Here's how the part is built. I have some questions about the finished solid (model axes, mm). A direction names the side the tool comes from. Round coordinates to 2 decimals unless told otherwise and drop trailing zeros. Write each loop counter-clockwise with the first axis right and the second up, starting at its lowest first coordinate (ties: lowest second). Pieces come first, ordered by that corner, then holes. Notation, with made-up numbers: (36.25, 22.5) -> (41.25, 22.5) arc R22 cw to (41.25, 45.5) -> close; hole circle Ø9 at (61.5, 7.25). An arc over 180 degrees is marked (long way). Put each result on its own line as item: value. Start each with the question number.
1) We'd pull the mould along X, two halves only. Please class faces 1 (the flat face through (27.254, -17, -25)), 2 (the flat face through (11.252, -17, -30)), 3 (the flat face through (31.254, -17, -25)): released by +X, released by -X, zero draft, split by the parting line, or undercut.
2) Which directions (+Z, -Z, +X, -X, +Y, -Y) give clear straight access to the entire face, cutting with the end or side of a thin tool? Please do faces 4 (the flat face through (3.308, -18, -25)), 5 (the flat face through (25.5, -15.6, -28.5)), 6 (the flat face through (7.3, -15.6, -28.5)), 7 (the flat face through (22.36, -17, -25)), 8 (the flat face through (16.678, -17.513, -30.305)).
3) I want a section at A-A, the plane x = 7.5. List the corners of the cut face in (y, z) for me, then the cut area to 3 significant figures.
4) If I drill on line 1 along X through (y, z) = (-17.5, -25.75); line 2 along Y through (x, z) = (23.5, -26.5); line 3 along X through (y, z) = (-18, -25.75), over which ranges is the centre line in solid material (lowest first)? Write a range as [from, to].
5) I want a section at D-D, the plane z = -23. List the corners of the cut face in (x, y) for me.
6) I want a section at C-C, the plane z = -30.25. List the corners of the cut face in (x, y) for me, then the cut area to 3 significant figures.
7) I want a section at B-B, the plane y = -20. List the corners of the cut face in (x, z) for me, then the cut area to 3 significant figures.
8) Will these pins go through, and if not, where does the flat tip stop? P1, Ø1.5, axis at y = -16, z = -30, coming from the -X side; P2, Ø2.5, axis at x = 8.5, y = -16.5, coming from the -Z side; P3, Ø2, axis at x = 16.058, z = -28.5, coming from the -Y side; P4, Ø2.5, axis at y = -16, z = -30.5, coming from the +X side.
Solid Edge part; units mm, degrees
sketch "Sketch1" plane through (0, 0, -22.5) normal (0, 0, 1) x (1, 0, 0)
  line L0 (22.3605, -19.157) -> (22.3605, -15.757)
  line L1 (22.3605, -15.757) -> (27.2537, -15.757)
  line L2 (27.2537, -15.757) -> (27.2537, -19.157)
  line L3 (27.2537, -19.157) -> (22.3605, -19.157)
  line L4 (3.308, -13.457) -> (31.2537, -13.457)
  line L5 (31.2537, -13.457) -> (31.2537, -21.457)
  line L6 (31.2537, -21.457) -> (3.308, -21.457)
  line L7 (3.308, -21.457) -> (3.308, -13.457)
  circle A0 centre (7.308, -17.457) radius 1.7
extrude "ExtrudedProtrusion_1" add sketch "Sketch1" against normal blind 9
sketch "Sketch2" plane through (17.2808, -21.457, -27.5) normal (0, -1, 0) x (0, 0, -1)
  line L0 (2.1809, 0) -> (3.4472, -1.2228)
  line L1 (3.4472, -1.2228) -> (2.1809, -2.4457)
  arc A0 (2.1809, -2.4457) -> (2.1809, 0) centre (1, -1.2228) cw
  dimension "D1" = 1
extrude "Cutout1" cut sketch "Sketch2" against normal up to next
sketch "Sketch3" plane through (17.2808, -17.457, -31.5) normal (0, 0, -1) x (0, 1, 0)
  line L0 (-9.6759, 16.4709) -> (6.2372, 16.4709)
  line L1 (6.2372, 16.4709) -> (6.2372, 2.6566)
  line L2 (6.2372, 2.6566) -> (-9.6759, 2.6566)
  line L3 (-9.6759, 2.6566) -> (-9.6759, 16.4709)
  line L4 (6.2372, -6.0293) -> (-9.6759, -6.0293)
  line L5 (-9.6759, -6.0293) -> (-9.6759, -15.1311)
  line L6 (-9.6759, -15.1311) -> (6.2372, -15.1311)
  line L7 (6.2372, -15.1311) -> (6.2372, -6.0293)
extrude "ExtrudedCutout_2" cut sketch "Sketch3" against normal blind 3
Findings:
1. face 1: undercut
1. face 2: released by -X
1. face 3: released by +X
2. face 4: +Z, -Z, -X, +Y, -Y
2. face 5: -Z, +X, +Y, -Y
2. face 6: -Z, -X, +Y, -Y
2. face 7: +Z, -Z
2. face 8: +Y, -Y
3. outline: (-21.46, -28.5) -> (-19.15, -28.5) -> (-19.15, -22.5) -> (-21.46, -22.5) -> close; (-15.77, -28.5) -> (-13.46, -28.5) -> (-13.46, -22.5) -> (-15.77, -22.5) -> close
3. area: 27.7 mm2
4. line 1: x = [3.31, 5.61], [9.01, 22.36], [27.25, 31.25]
4. line 2: y = [-21.46, -19.16], [-15.76, -13.46]
4. line 3: x = [3.31, 5.7], [8.92, 22.36], [27.25, 31.25]
5. outline: (3.31, -21.46) -> (31.25, -21.46) -> (31.25, -13.46) -> (3.31, -13.46) -> close; hole circle Ø3.4 at (7.31, -17.46); hole (22.36, -19.16) -> (27.25, -19.16) -> (27.25, -15.76) -> (22.36, -15.76) -> close
6. outline: (11.25, -21.46) -> (15.38, -21.46) -> (15.38, -13.46) -> (11.25, -13.46) -> close; (16.73, -21.46) -> (19.94, -21.46) -> (19.94, -13.46) -> (16.73, -13.46) -> close
6. area: 58.7 mm2
7. outline: (3.31, -28.5) -> (11.25, -28.5) -> (11.25, -31.5) -> (19.94, -31.5) -> (19.94, -28.5) -> (31.25, -28.5) -> (31.25, -22.5) -> (3.31, -22.5) -> close; hole (14.84, -29.68) -> (16.06, -30.95) -> (17.28, -29.68) arc R1.7 ccw (long way) to start
7. area: 184 mm2
8. P1: stops at x = 11.25
8. P2: stops at z = -28.5
8. P3: passes through
8. P4: stops at x = 19.94
